Here's how the part is built. I have some questions about the finished solid (model axes, mm). Round coordinates to 2 decimals unless told otherwise and drop trailing zeros. Order: outer loops, then holes, each group sorted by start corner. A loop starts at its lowest first (then second) coordinate and runs counter-clockwise, first axis right, second up. Notation, with made-up numbers: (19.25, 17) -> (66.25, 17) arc R26 cw to (66.25, 51) -> close; hole circle Ø1 at (51.5, -30.75). An arc over 180 degrees is marked (long way). One line per item, written item: value.
```python
from build123d import *

# Parameters (mm, degrees)
BOSS_EXTRUDE1_DEPTH = 0.5
SKETCH2_R           = 1.5
CUT_EXTRUDE1_DEPTH  = 0.5
SKETCH3_R           = 1.5
CUT_EXTRUDE2_DEPTH  = 0.5
SKETCH4_W           = 22
SKETCH4_H           = 5
CUT_EXTRUDE3_DEPTH  = 0.5


with BuildPart() as part:
    # Sketch1 → Boss-Extrude1 (new body)
    with BuildSketch(Plane.XY):
        with BuildLine():
            Line((0, 4.666666667), (28, 4.666666667))
            ThreePointArc((28, 4.666666667), (32.666666667, 0), (28, -4.666666667))
            Line((28, -4.666666667), (0, -4.666666667))
            ThreePointArc((0, -4.666666667), (-4.666666667, 0), (0, 4.666666667))
        make_face()
    extrude(amount=BOSS_EXTRUDE1_DEPTH)

    # Sketch2 → Cut-Extrude1 (cut)
    with BuildSketch(Plane.XY.offset(0.5)):
        Circle(SKETCH2_R)
    extrude(amount=-CUT_EXTRUDE1_DEPTH, mode=Mode.SUBTRACT)

    # Sketch3 → Cut-Extrude2 (cut)
    with BuildSketch(Plane.XY.offset(0.5)):
        with Locations((28, 0)):
            Circle(SKETCH3_R)
    extrude(amount=-CUT_EXTRUDE2_DEPTH, mode=Mode.SUBTRACT)

    # Sketch4 → Cut-Extrude3 (cut)
    with BuildSketch(Plane.XY.offset(0.5)):
        with Locations((14, 0)):
            Rectangle(SKETCH4_W, SKETCH4_H)
    extrude(amount=-CUT_EXTRUDE3_DEPTH, mode=Mode.SUBTRACT)


solid = part.part
```
Q1. If we mould it in two halves opening along X, with no side actions, what happens to faces 1 (the face through (32.666, 0.103, 0.246)), 2 (the face through (26.5, 0.07, 0.25)), 3 (the face through (14, -3, 0)), 4 (the face through (-4.666, -0.103, 0.246))? For each: pulls with the +X half, pulls with the -X half, needs draft (parallel to the pull), parting line crosses it, or undercut.
Answers:
face 1: pulls with the +X half
face 2: undercut
face 3: needs draft
face 4: pulls with the -X half
Q2. I want a section at D-D on x = 29. Write out the boundary of the cut face in (y, z), then the cut area to 3 significant figures.
Answers:
outline: (-4.56, 0) -> (-1.12, 0) -> (-1.12, 0.5) -> (-4.56, 0.5) -> close; (1.12, 0) -> (4.56, 0) -> (4.56, 0.5) -> (1.12, 0.5) -> close
area: 3.44 mm2
Q3. I want a section at B-B on x = 6. Write out the boundary of the cut face in (y, z), then the cut area to 3 significant figures.
Answers:
outline: (-4.67, 0) -> (-2.5, 0) -> (-2.5, 0.5) -> (-4.67, 0.5) -> close; (2.5, 0) -> (4.67, 0) -> (4.67, 0.5) -> (2.5, 0.5) -> close
area: 2.17 mm2
Q4. I need wall thicknesses on line 1 along Y through (x, z) = (28, 0.25); line 2 along Y through (x, z) = (22, 0.1); line 3 along X through (y, z) = (-1, 0.3). Which ranges of each line are inside material? Lowest first, please.
Answers:
line 1: -4.67 to -1.5, 1.5 to 4.67
line 2: -4.67 to -2.5, 2.5 to 4.67
line 3: -4.56 to -1.12, 1.12 to 3, 25 to 26.88, 29.12 to 32.56
Q5. I want a section at C-C on z = 0.2. Write out the boundary of the cut face in (x, y).
Answers:
outline: (0, -4.67) -> (28, -4.67) arc R4.67 ccw to (28, 4.67) -> (0, 4.67) arc R4.67 ccw to start; hole circle Ø3 at (0, 0); hole (3, -2.5) -> (25, -2.5) -> (25, 2.5) -> (3, 2.5) -> close; hole circle Ø3 at (28, 0)
Q6. I want a section at A-A on y = 0. Write out the boundary of the cut face in (x, z).
Answers:
outline: (-4.67, 0) -> (-1.5, 0) -> (-1.5, 0.5) -> (-4.67, 0.5) -> close; (1.5, 0) -> (3, 0) -> (3, 0.5) -> (1.5, 0.5) -> close; (25, 0) -> (26.5, 0) -> (26.5, 0.5) -> (25, 0.5) -> close; (29.5, 0) -> (32.67, 0) -> (32.67, 0.5) -> (29.5, 0.5) -> close
